The model under review builds one solid part; all positions refer to its coordinate system, in mm. A direction names the side the tool comes from. Round coordinates to 2 decimals unless told otherwise and drop trailing zeros. Order: outer loops, then holes, each group sorted by start corner. A loop starts at its lowest first (then second) coordinate and runs counter-clockwise, first axis right, second up.
Autodesk Inventor part; units mm, degrees
ref_plane "YZ Plane" through (0, 0, 0) normal (1, 0, 0) x (0, 1, 0)
ref_plane "XZ Plane" through (0, 0, 0) normal (0, 1, 0) x (-1, 0, 0)
ref_plane "XY Plane" through (0, 0, 0) normal (0, 0, 1) x (1, 0, 0)
sketch "Sketch1" plane through (0, 0, 0) normal (0, 1, 0) x (-1, 0, 0)
  line L0 (2.3094, 4) -> (4.6188, 0)
  line L1 (4.6188, 0) -> (2.3094, -4)
  line L2 (2.3094, -4) -> (-2.3094, -4)
  line L3 (-2.3094, -4) -> (-4.6188, 0)
  line L4 (-4.6188, 0) -> (-2.3094, 4)
  line L5 (-2.3094, 4) -> (2.3094, 4)
  line L6 (4.6188, -8) -> (9.2376, 0)
  line L7 (9.2376, 0) -> (4.6188, 8)
  line L8 (4.6188, 8) -> (-4.6188, 8)
  line L9 (-4.6188, 8) -> (-9.2376, 0)
  line L10 (-9.2376, 0) -> (-4.6188, -8)
  line L11 (-4.6188, -8) -> (4.6188, -8)
  point P0 (0, 0)
  point P1 (0, 0)
  dimension "d1" = 8
  dimension "d2" = 4
extrude "Extrusion1" add sketch "Sketch1" along normal blind 5.9531
sketch "Sketch2" plane through (0, 5.9531, 0) normal (0, 1, 0) x (1, 0, 0)
  circle A0 centre (0, 0) radius 19.2376
  line L0 (4.6188, -8) -> (9.2376, 0)
  circle A1 centre (0, 0) radius 9.2376
  dimension "d5" = 10
extrude "Extrusion2" add sketch "Sketch2" along normal blind 5 contours A0 | A1 L0 | L0 A1
sketch "Sketch3" plane through (0, 0, 0) normal (0, -1, 0) x (1, 0, 0)
  line L0 (4.6188, -8) -> (-4.6188, -8)
  line L1 (0, -8) -> (2.5, -8)
  line L2 (0, -8) -> (-2.5, -8)
  line L3 (2.5, -8) -> (-2.5, -8)
  line L4 (-2.5, -8) -> (-2.5, -28)
  line L5 (-2.5, -28) -> (2.5, -28)
  line L6 (2.5, -28) -> (2.5, -8)
  point P0 (0, 0)
  dimension "d8" = 2.5
  dimension "d9" = 2.5
  dimension "d10" = 20
extrude "Extrusion3" add sketch "Sketch3" against normal up to surface (10.9531 mm away)
properties part number "wingnut"
(1) Consider section D-D (y = 6.5). Write out the cut boundary in (x, z).
Data:
outline: (-2.5, -28) - (2.5, -28) - (2.5, -19.07) arc R19.24 ccw (long way) to (-2.5, -19.07) - close
(2) Consider section B-B (x = 0). Write out the cut boundary in (y, z).
Data:
outline: (0, -28) - (10.95, -28) - (10.95, 19.24) - (5.95, 19.24) - (5.95, 8) - (0, 8) - (0, 4) - (5.95, 4) - (5.95, -4) - (0, -4) - close
(3) To check wall thickness, follow probe 1 along Z at (x, y) = (0.5, 3.5); probe 2 along Y at (x, z) = (2, 12); probe 3 along X at (y, z) = (4.5, -16). State the ranges of each line that lie inside material, in increasing order.
Data:
probe 1: z = -28 to -4, 4 to 8
probe 2: y = 5.95 to 10.95
probe 3: x = -2.5 to 2.5
(4) Draft analysis for pull direction X (two halves, no side actions). For faces 4 (the flat face through (0, 10.953, 1)), 5 (the flat face through (-6.896, 2.935, -4.056)), 6 (the flat face through (0, 5.953, 0)), 7 (the flat face through (0, 3, 4)), state which applies: pulls with the +X half, pulls with the -X half, needs draft (parallel to the pull), parting line crosses it, or undercut.
Data:
face 4: needs draft
face 5: pulls with the -X half
face 6: undercut
face 7: undercut
(5) Consider section A-A (y = 2.75). Write out the cut boundary in (x, z).
Data:
outline: (-9.24, 0) - (-4.62, -8) - (-2.5, -8) - (-2.5, -28) - (2.5, -28) - (2.5, -8) - (4.62, -8) - (9.24, 0) - (4.62, 8) - (-4.62, 8) - close; hole (-4.62, 0) - (-2.31, -4) - (2.31, -4) - (4.62, 0) - (2.31, 4) - (-2.31, 4) - close
(6) Consider section C-C (z = -22.5). Write out the cut boundary in (x, y), and give its area (3 significant figures).
Data:
outline: (-2.5, 0) - (2.5, 0) - (2.5, 10.95) - (-2.5, 10.95) - close
area: 54.8 mm2
(7) For faces 1 (the flat face through (6.896, 2.935, 4.056)), 2 (the flat face through (6.961, 2.935, -3.944)), 3 (the flat face through (0, 3, 8)), list the 3-axis set-ups (+Z, -Z, +X, -X, +Y, -Y) from which the entire face can be reached by the end or side of a thin tool; tool diameter is ignored.
Data:
face 1: +Z, +X, -Y
face 2: -Z, +X, -Y
face 3: +Z, +X, -X, -Y
(8) Insertion check: pin 1 (2 mm diameter, centred on x = -6, y = 2.5, fed in from +Z); pin 2 (3 mm diameter, centred on x = -10, y = 9, fed in from -Z); pin 3 (1.7 mm diameter, centred on x = -4, y = 3, fed in from -Z). Each pin has a flat end and moves straight along its axis. Give the tip position at first contact, or say it passes through.
Data:
pin 1: stops at z = 7.34
pin 2: stops at z = -17.26
pin 3: stops at z = -8
